Drawing for the job (mm, zero at the part's lowest x, y, z). Round coordinates to 2 decimals unless told otherwise and drop trailing zeros. Write each loop counter-clockwise with the first axis right and the second up, starting at its lowest first coordinate (ties: lowest second). Pieces come first, ordered by that corner, then holes.
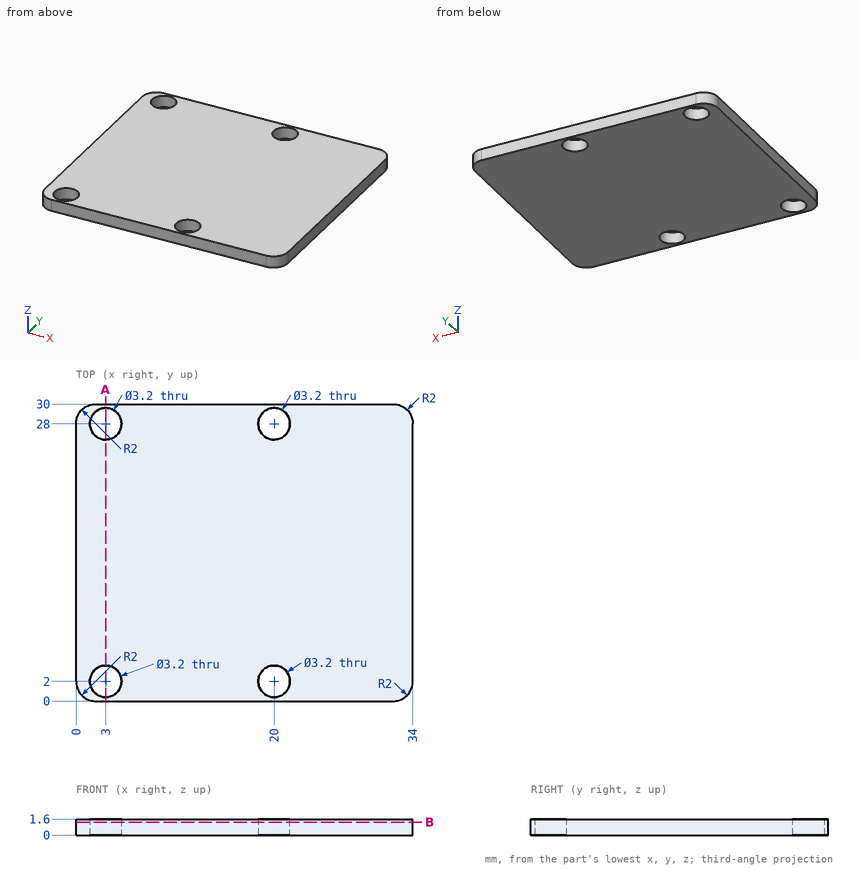
1) Cut at A-A on x = 3. List the corners of the cut face in (y, z).
2) Cut at B-B on z = 1.3. List the corners of the cut face in (x, y).
3) Flat gauge pin, fed straight in: pin 1 Ø2.5 at (x, y) = (20, 2) entering from +Z. Where does the tip first touch, or does it go through?
4) Wall check: probe 1 along X at (y, z) = (2, 1.25); probe 2 along Y at (x, z) = (20, 0.7); probe 3 along Y at (x, z) = (2.5, 1.55). Give the ranges that are in metal, low to high.
Result sheet:
1. outline: (0, 0) - (0.4, 0) - (0.4, 1.6) - (0, 1.6) - close; (3.6, 0) - (26.4, 0) - (26.4, 1.6) - (3.6, 1.6) - close; (29.6, 0) - (30, 0) - (30, 1.6) - (29.6, 1.6) - close
2. outline: (0, 2) arc R2 ccw to (2, 0) - (32, 0) arc R2 ccw to (34, 2) - (34, 28) arc R2 ccw to (32, 30) - (2, 30) arc R2 ccw to (0, 28) - close; hole circle Ø3.2 at (3, 2); hole circle Ø3.2 at (3, 28); hole circle Ø3.2 at (20, 2); hole circle Ø3.2 at (20, 28)
3. pin 1: passes through
4. probe 1: x = 0 to 1.4, 4.6 to 18.4, 21.6 to 34
4. probe 2: y = 0 to 0.4, 3.6 to 26.4, 29.6 to 30
4. probe 3: y = 0 to 0.48, 3.52 to 26.48, 29.52 to 30
